Verification items for the finished model (mm, model axes). A direction names the side the tool comes from. Coordinates: 2 decimals unless noted, no trailing zeros. Loops run counter-clockwise (first coordinate to the right, second up) from the corner with the lowest first, then second, coordinate; pieces in that order, holes last.
Q1. Sectioned sample at D-D (z = 1.7). Count the separate pieces of the cut face and the enclosed holes in it, then the cut area to 3 significant figures.
Q2. Material ranges on probe 1 along Y at (x, z) = (6.35, 1.55) (3 decimals); probe 2 along Y at (x, z) = (3.25, 0.3) (3 decimals); probe 3 along Y at (x, z) = (16.25, 2), recorded low to high.
Q3. Mould release check, pull along X, two halves, no side actions. Record for faces 4 (the face through (6, 3.175, 1)), 5 (the face through (2.758, 23.697, 1.481)), 6 (the face through (2.147, 25.86, 1.481)), 7 (the face through (12.7, 5, 1)): +X half, -X half, draft (parallel to the pull), parting line (faces both ways), or undercut.
Q4. Sectioned sample at B-B (y = 12.7). Enter the section's corners in (x, z), then the cut area to 3 significant figures.
Q5. Access from +Z, -Z, +X, -X, +Y, -Y to the whole of each face (thin tool, end or side, straight path). Record for faces 1 (the face through (17.46, 4.53, 1.48)), 2 (the face through (13, 0, 1)), 3 (the face through (6, 6.096, 1)).
Q6. Sectioned sample at A-A (x = 6.35). Enter the section's corners in (y, z) (3 decimals), then the cut area to 3 significant figures.
Q7. Sectioned sample at C-C (y = 26). Enter the section's corners in (x, z).
Autodesk Inventor part; units mm, degrees
ref_plane "YZ Plane" through (0, 0, 0) normal (1, 0, 0) x (0, 1, 0)
ref_plane "XZ Plane" through (0, 0, 0) normal (0, 1, 0) x (-1, 0, 0)
ref_plane "XY Plane" through (0, 0, 0) normal (0, 0, 1) x (1, 0, 0)
sketch "Sketch1" plane through (0, 0, 0) normal (0, 0, 1) x (1, 0, 0)
  line L0 (0, 0) -> (25.4, 0)
  line L1 (25.4, 0) -> (25.4, 31.75)
  line L2 (25.4, 31.75) -> (0, 31.75)
  line L3 (0, 31.75) -> (0, 0)
  circle A0 centre (6.35, 12.7) radius 1.7882
  arc A1 (16.2884, 4.7932) -> (2.0063, 24.6341) centre (6.35, 12.7) ccw construction
  line L4 (2.5493, 23.1423) -> (1.4634, 26.1259)
  line L5 (6.35, 12.7) -> (20.6125, 12.7) construction
  arc A2 (15.0461, 5.7815) -> (2.5493, 23.1423) centre (6.35, 12.7) ccw
  arc A3 (17.5307, 3.8048) -> (1.4634, 26.1259) centre (6.35, 12.7) ccw
  line L6 (15.0461, 5.7815) -> (17.5307, 3.8048)
  dimension "d0" = 12.7
  dimension "d1" = 31.75
  dimension "d2" = 6.35
  dimension "d3" = 110
  dimension "d4" = 25.4
  dimension "d5" = 1.5875
  dimension "d6" = 1.5875
  dimension "d10" = 25.4
extrude "Extrusion1" add sketch "Sketch1" along normal blind 2.921
fillet "Fillet1" radius 1.5875 4 edges at (15.0461, 5.7815, 1.4605) (17.5307, 3.8048, 1.4605) (1.4634, 26.1259, 1.4605) (2.5493, 23.1423, 1.4605)
sketch "Sketch2" plane through (0, 0, 2.921) normal (0, 0, 1) x (1, 0, 0)
  line L0 (0, 3.175) -> (12.7, 3.175)
  line L1 (12.7, 3.175) -> (12.7, 6.096)
  line L2 (12.7, 6.096) -> (0, 6.096)
  line L3 (0, 6.096) -> (0, 3.175)
  line L4 (0, 0) -> (25.4, 0)
  line L5 (0, 31.75) -> (0, 0)
  dimension "d11" = 2.921
  dimension "d12" = 12.7
  dimension "d13" = 3.175
  dimension "d14" = 0
extrude "Extrusion2" cut sketch "Sketch2" against normal blind 6.604
fillet "Fillet2" radius 6.35 1 edges at (25.4, 31.75, 1.4605)
properties part number "Angleframe"
Geometry check:
1. separate pieces: 1
1. enclosed holes: 2
1. area: 648 mm2
2. probe 1: y = 0 to 3.175, 6.096 to 10.912, 14.488 to 23.812, 26.988 to 31.75
2. probe 2: y = 0 to 3.175, 6.096 to 23.521, 26.647 to 31.75
2. probe 3: y = 0 to 4.82, 7.65 to 17.75, 23 to 31.75
3. face 4: draft
3. face 5: undercut
3. face 6: undercut
3. face 7: -X half
4. outline: (0, 0) - (4.56, 0) - (4.56, 2.92) - (0, 2.92) - close; (8.14, 0) - (17.46, 0) - (17.46, 2.92) - (8.14, 2.92) - close; (20.64, 0) - (25.4, 0) - (25.4, 2.92) - (20.64, 2.92) - close
4. area: 54.5 mm2
5. face 1: +Z, -Z
5. face 2: +Z, -Z, +X, -X, -Y
5. face 3: +Z, -Z, -X
6. outline: (0, 0) - (3.175, 0) - (3.175, 2.921) - (0, 2.921) - close; (6.096, 0) - (10.912, 0) - (10.912, 2.921) - (6.096, 2.921) - close; (14.488, 0) - (23.812, 0) - (23.812, 2.921) - (14.488, 2.921) - close; (26.988, 0) - (31.75, 0) - (31.75, 2.921) - (26.988, 2.921) - close
6. area: 64.5 mm2
7. outline: (0, 0) - (2.24, 0) - (2.24, 2.92) - (0, 2.92) - close; (11.57, 0) - (25.37, 0) - (25.37, 2.92) - (11.57, 2.92) - close
